CAD build for the part. Positions are in the model's coordinates, mm. Coordinates: 2 decimals unless noted, no trailing zeros. Order: outer loops, then holes, each group sorted by start corner. A loop starts at its lowest first (then second) coordinate and runs counter-clockwise, first axis right, second up. Notation, with made-up numbers: M 39,3.25 L 49,3.25 A11 cw 49,20.25 Z; hole C 54,47 d3. An arc over 180 degrees is marked long. Write item = value, one per line.
Autodesk Inventor part; units mm, degrees
ref_plane "YZ Plane" through (0, 0, 0) normal (1, 0, 0) x (0, 1, 0)
ref_plane "XZ Plane" through (0, 0, 0) normal (0, 1, 0) x (-1, 0, 0)
ref_plane "XY Plane" through (0, 0, 0) normal (0, 0, 1) x (1, 0, 0)
sketch "Sketch1" plane through (0, 0, 0) normal (0, 0, 1) x (1, 0, 0)
  circle A0 centre (0, 0) radius 1.5
  arc A1 (53.9189, 18.4865) -> (-57, 0) centre (0, 0) ccw
  arc A2 (55, 12) -> (53.9189, 18.4865) centre (35, 12) ccw
  line L0 (55, 12) -> (55, -11)
  line L1 (55, -11) -> (52, -11)
  line L2 (52, -11) -> (52, -23)
  line L3 (52, -23) -> (54.739, -23)
  line L4 (54.739, -23) -> (42, -58)
  line L5 (42, -58) -> (-57, -58)
  line L6 (-57, -58) -> (-57, -23)
  line L7 (-57, -23) -> (-51, -23)
  line L8 (-51, -23) -> (-51, -11)
  line L9 (-51, -11) -> (-57, -11)
  line L10 (-57, 0) -> (-57, -11)
  dimension "d0" = 3
  dimension "d1" = 57
  dimension "d2" = 20
  dimension "d3" = 6
  dimension "d4" = 12
  dimension "d5" = 55
  dimension "d6" = 3
  dimension "d7" = 110
  dimension "d8" = 99
  dimension "d9" = 47
  dimension "d10" = 58
extrude "Extrusion1" add sketch "Sketch1" along normal blind 1.5
fillet "Fillet1" radius 0.5 4 edges at (52, -11, 0.75) (52, -23, 0.75) (-51, -11, 0.75) (-51, -23, 0.75)
fillet "Fillet2" radius 1 4 edges at (-57, -11, 0.75) (-57, -23, 0.75) (54.739, -23, 0.75) (55, -11, 0.75)
fillet "Fillet3" radius 5 2 edges at (42, -58, 0.75) (-57, -58, 0.75)
properties part number "PT Flange Outer"
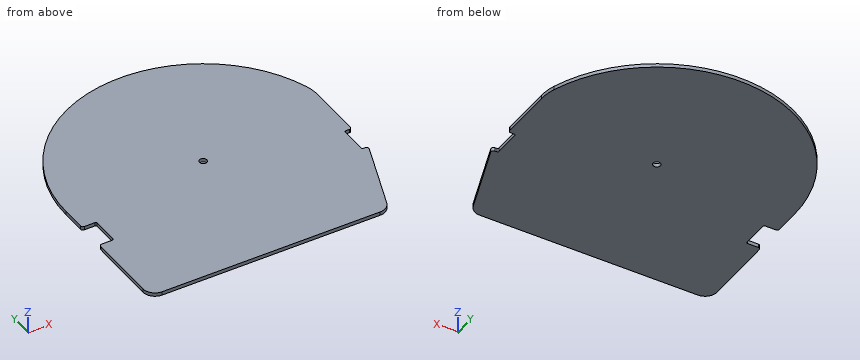
(1) Wall check: line 1 (Y direction, x = 0, z = 1.25); line 2 (Y direction, x = -42, z = 0.7); line 3 (Y direction, x = 8, z = 1.25). Give the ranges that are in metal, low to high. Write a range as from..to.
Evaluation:
line_1 = -58..-1.5, 1.5..57
line_2 = -58..38.54
line_3 = -58..56.44
(2) Slice it at C-C, the plane y = 27.5. Write the cut outline in (x, z).
Evaluation:
outline = M -49.93,0 L 49.93,0 L 49.93,1.5 L -49.93,1.5 Z
(3) Slice it at A-A, the plane x = 0. Write the cut outline in (y, z), then the cut area to 3 significant figures.
Evaluation:
outline = M -58,0 L -1.5,0 L -1.5,1.5 L -58,1.5 Z; M 1.5,0 L 57,0 L 57,1.5 L 1.5,1.5 Z
area = 168 mm²
(4) Slice it at D-D, the plane x = 14. Write the cut outline in (y, z), then the cut area to 3 significant figures.
Evaluation:
outline = M -58,0 L 55.25,0 L 55.25,1.5 L -58,1.5 Z
area = 170 mm²
(5) Slice it at B-B, the plane z = 0.95. Write the cut outline in (x, y), then the cut area to 3 significant figures.
Evaluation:
outline = M -57,-53 A5 ccw -52,-58 L 38.5,-58 A5 ccw 43.2,-54.71 L 54.25,-24.34 A1 ccw 53.31,-23 L 52.5,-23 A0.5 cw 52,-22.5 L 52,-11.5 A0.5 cw 52.5,-11 L 54,-11 A1 ccw 55,-10 L 55,12 A20 ccw 53.92,18.49 A57 ccw -57,0 L -57,-10 A1 ccw -56,-11 L -51.5,-11 A0.5 cw -51,-11.5 L -51,-22.5 A0.5 cw -51.5,-23 L -56,-23 A1 ccw -57,-24 Z; hole C 0,0 d3
area = 11,200 mm²
(6) Pin check, flat tip, straight feed: pin 1 Ø0.6 at (x, z) = (53, 1) entering from +Y. Stop position of the tip, or through.
Evaluation:
pin_1 = 21.72
